Part model, mm, in its own coordinate system. A direction names the side the tool comes from. Give positions to 0.01 mm unless a question says otherwise; leave off trailing zeros. Write each loop counter-clockwise with the first axis right and the second up, starting at its lowest first coordinate (ties: lowest second). Pieces come first, ordered by that corner, then holes. Notation, with made-up numbers: M 27.25,20 L 54.25,20 A5 ccw 54.25,26 Z; hole C 45.25,-27 d3. An arc over 180 degrees is marked long. Answer as CSV lines item,"result". Start each with the question number.
Item 1: 3-axis set-ups, long thin cutter, end or side, ignore diameter. For faces 1 (the cylindrical face through (-7.02, 21.23, 1.52)), 2 (the flat face through (7, 9, 2)), 3 (the flat face through (-7, -29, 2)): which of +Z, -Z, +X, -X, +Y, -Y reach the whole face in a straight line?
Item 2: Pin check, flat tips, straight feed: pin 1 (0.7 mm diameter, centred on x = -9.5, z = 1, fed in from -Y); pin 2 (0.9 mm diameter, centred on y = 27.5, z = 1.5, fed in from +X); pin 3 (0.7 mm diameter, centred on x = -9.5, z = 1, fed in from +Y). Stop position of each tip, or through.
Item 3: Wall check: L1, parallel to Y at x = 8.25, z = 2.6; L2, parallel to X at y = 21, z = 2.9; L3, parallel to X at y = -27, z = 0.7. Give the ranges that are in metal, low to high. Write a range as from..to.
Item 4: Band-saw the part on A-A, the plane y = 24. List the corners of the cut face in (x, z), then the cut area to 3 significant figures.
Item 5: Two-plate mould, pull along Y, no slides. Class faces 4 (the flat face through (0, 0, 3)), 5 (the flat face through (0, 35, 1)), 6 (the flat face through (-7, -9, 2)), 7 (the cylindrical face through (-6.98, -21.27, 1.52)): +Y half, -Y half, draft (parallel to the pull), parting line (faces both ways), or undercut.
Item 6: Band-saw the part on B-B, the plane y = -3.5. List the corners of the cut face in (x, z), then the cut area to 3 significant figures.
from build123d import *

# Parameters (mm, degrees)
CROQUIS1_W              = 20
CROQUIS1_H              = 70
SALIENTE_EXTRUIR1_DEPTH = 3
CROQUIS2_W              = 3
CROQUIS2_H              = 13.75
CORTAR_EXTRUIR1_DEPTH   = 4
CROQUIS3_R              = 1.5
CORTAR_EXTRUIR2_DEPTH   = 4


with BuildPart() as part:
    # Croquis1 → Saliente-Extruir1 (new body)
    with BuildSketch(Plane.XY):
        Rectangle(CROQUIS1_W, CROQUIS1_H)
    extrude(amount=SALIENTE_EXTRUIR1_DEPTH)

    # Croquis2 → Cortar-Extruir1 (cut, through all)
    with BuildSketch(Plane.XY.offset(3)):
        with Locations((8.5, 28.125)):
            Rectangle(CROQUIS2_W, CROQUIS2_H)
        with Locations((8.5, 9.375)):
            Rectangle(CROQUIS2_W, CROQUIS2_H)
        with Locations((8.5, -28.125)):
            Rectangle(CROQUIS2_W, CROQUIS2_H)
        with Locations((8.5, -9.375)):
            Rectangle(CROQUIS2_W, CROQUIS2_H)
        with Locations((-8.5, -9.375)):
            Rectangle(CROQUIS2_W, CROQUIS2_H)
        with Locations((-8.5, -28.125)):
            Rectangle(CROQUIS2_W, CROQUIS2_H)
        with Locations((-8.5, 9.375)):
            Rectangle(CROQUIS2_W, CROQUIS2_H)
        with Locations((-8.5, 28.125)):
            Rectangle(CROQUIS2_W, CROQUIS2_H)
    extrude(amount=-CORTAR_EXTRUIR1_DEPTH, mode=Mode.SUBTRACT)

    # Croquis3 → Cortar-Extruir2 (cut, through all)
    with BuildSketch(Plane.XY.offset(3)):
        with Locations((8.060660172, 22.310660172)):
            Circle(CROQUIS3_R)
        with Locations((8.060660172, 15.189339828)):
            Circle(CROQUIS3_R)
        with Locations((8.060660172, 3.560660172)):
            Circle(CROQUIS3_R)
        with Locations((8.060660172, -3.560660172)):
            Circle(CROQUIS3_R)
        with Locations((8.060660172, -15.189339828)):
            Circle(CROQUIS3_R)
        with Locations((8.060660172, -22.310660172)):
            Circle(CROQUIS3_R)
        with Locations((-8.060660172, -22.310660172)):
            Circle(CROQUIS3_R)
        with Locations((-8.060660172, -15.189339828)):
            Circle(CROQUIS3_R)
        with Locations((-8.060660172, -3.560660172)):
            Circle(CROQUIS3_R)
        with Locations((-8.060660172, 3.560660172)):
            Circle(CROQUIS3_R)
        with Locations((-8.060660172, 15.189339828)):
            Circle(CROQUIS3_R)
        with Locations((-8.060660172, 22.310660172)):
            Circle(CROQUIS3_R)
    extrude(amount=-CORTAR_EXTRUIR2_DEPTH, mode=Mode.SUBTRACT)


solid = part.part
Output:
1,face 1,"+Z, -Z"
1,face 2,"+Z, -Z, +X"
1,face 3,"+Z, -Z, -X, -Y"
2,pin 1,"y = -21.25"
2,pin 2,"x = 7"
2,pin 3,"y = 21.25"
3,L1,"-20.82..-16.68, -2.07..2.07, 16.68..20.82"
3,L2,"-10..-8.79, -7.33..7.33, 8.79..10"
3,L3,"-7..7"
4,outline,"M -7,0 L 7,0 L 7,3 L -7,3 Z"
4,area,"42.0 mm²"
5,face 4,"draft"
5,face 5,"+Y half"
5,face 6,"undercut"
5,face 7,"undercut"
6,outline,"M -6.56,0 L 6.56,0 L 6.56,3 L -6.56,3 Z"
6,area,"39.4 mm²"
